```python
from build123d import *

# Parameters (mm, degrees)
SKETCH1_W           = 72
SKETCH1_H           = 47
SKETCH1_W_2         = 5
SKETCH1_H_2         = 13.68224698
SKETCH1_H_3         = 13
BOSS_EXTRUDE1_DEPTH = 5
SKETCH3_W           = 14.035397612
SKETCH3_H           = 7.623801165
BOSS_EXTRUDE3_DEPTH = 5
SKETCH5_W           = 14.035397612
SKETCH5_H           = 7.623801165
BOSS_EXTRUDE4_DEPTH = 5
SKETCH4_R           = 1.799999998
CUT_EXTRUDE1_DEPTH  = 95
SKETCH6_W           = 72
SKETCH6_H           = 5
BOSS_EXTRUDE5_DEPTH = 21
SKETCH8_W           = 114.485355007
SKETCH8_H           = 45.141194617
CUT_EXTRUDE2_DEPTH  = 4.5
SKETCH9_W           = 62
SKETCH9_H           = 5
CUT_EXTRUDE3_DEPTH  = 4.5


with BuildPart() as part:
    # Sketch1 → Boss-Extrude1 (new body)
    with BuildSketch(Plane(origin=(0, 0, 0), x_dir=(1, 0, 0), z_dir=(0, 1, 0))):
        with Locations((36, -23.5)):
            Rectangle(SKETCH1_W, SKETCH1_H)
        with Locations((69.5, 6.84112349)):
            Rectangle(SKETCH1_W_2, SKETCH1_H_2)
        with Locations((2.5, 6.5)):
            Rectangle(SKETCH1_W_2, SKETCH1_H_3)
    extrude(amount=BOSS_EXTRUDE1_DEPTH)

    # Sketch3 → Boss-Extrude3 (add)
    with BuildSketch(Plane(origin=(72, 0, 0), x_dir=(0, 0, -1), z_dir=(1, 0, 0))):
        with Locations((6.664548174, 1.188099417)):
            Rectangle(SKETCH3_W, SKETCH3_H)
    extrude(amount=-BOSS_EXTRUDE3_DEPTH)

    # Sketch5 → Boss-Extrude4 (add)
    with BuildSketch(Plane.ZY):
        with Locations((-6.664548174, 1.188099417)):
            Rectangle(SKETCH5_W, SKETCH5_H)
    extrude(amount=-BOSS_EXTRUDE4_DEPTH)

    # Sketch4 → Cut-Extrude1 (cut)
    with BuildSketch(Plane(origin=(72, 0, 0), x_dir=(0, 0, -1), z_dir=(1, 0, 0))):
        with Locations((4.182640247, 1.972422216)):
            Circle(SKETCH4_R)
    extrude(amount=-CUT_EXTRUDE1_DEPTH, mode=Mode.SUBTRACT)

    # Sketch6 → Boss-Extrude5 (add)
    with BuildSketch(Plane.XY.offset(47)):
        with Locations((36, 2.5)):
            Rectangle(SKETCH6_W, SKETCH6_H)
    extrude(amount=BOSS_EXTRUDE5_DEPTH)

    # Sketch8 → Cut-Extrude2 (cut)
    with BuildSketch(Plane(origin=(0, 0, -13.68224698), x_dir=(-1, 0, 0), z_dir=(0, 0, -1))):
        with Locations((-40.6465034, -1.597733879)):
            Rectangle(SKETCH8_W, SKETCH8_H)
    extrude(amount=-CUT_EXTRUDE2_DEPTH, mode=Mode.SUBTRACT)

    # Sketch9 → Cut-Extrude3 (cut)
    with BuildSketch(Plane(origin=(0, 0, 0), x_dir=(-1, 0, 0), z_dir=(0, 0, -1))):
        with Locations((-36, 2.5)):
            Rectangle(SKETCH9_W, SKETCH9_H)
    extrude(amount=-CUT_EXTRUDE3_DEPTH, mode=Mode.SUBTRACT)


solid = part.part
```
Work out the finished part from the listing and answer in its coordinate system (mm). A direction names the side the tool comes from. Give positions to 0.01 mm unless a question says otherwise; leave off trailing zeros. Order: outer loops, then holes, each group sorted by start corner. A loop starts at its lowest first (then second) coordinate and runs counter-clockwise, first axis right, second up.
1. For faces 4 (the flat face through (35, 3, 68)), 5 (the flat face through (35, 0, 34)), 6 (the flat face through (36, 3, 4.5)), determine the directions among +Z, -Z, +X, -X, +Y, -Y from which every point of the face is accessible in a straight line to the end or side of a thin tool.
Result sheet:
face 4: +Z, +X, -X, +Y, -Y
face 5: +Z, +X, -X, -Y
face 6: -Z, +Y, -Y
2. Section A-A, the plane y = -1.5 is taken. Determine the outline of the cut face in (x, z), and give its area (3 significant figures).
Result sheet:
outline: (0, -9.18) - (5, -9.18) - (5, 0.35) - (0, 0.35) - close; (67, -9.18) - (72, -9.18) - (72, 0.35) - (67, 0.35) - close
area: 95.4 mm2
3. Section B-B, the plane x = 6 is taken. Determine the outline of the cut face in (y, z).
Result sheet:
outline: (0, 4.5) - (5, 4.5) - (5, 68) - (0, 68) - close
4. Section C-C, the plane z = 7 is taken. Determine the outline of the cut face in (x, y).
Result sheet:
outline: (0, 0) - (72, 0) - (72, 5) - (0, 5) - close
5. Straight lines are drawn through the part: L1, parallel to Y at x = 20, z = 19; L2, parallel to Z at x = 43, y = 4.5; L3, parallel to Z at x = 4.5, y = 3.5. For each, find the intervals that lie inside material, in ascending order.
Result sheet:
L1: y = 0 to 5
L2: z = 4.5 to 68
L3: z = -9.18 to -5.13, -3.23 to 68
6. Each of these flat-tipped pins is pushed along its axis until it touches: P1, Ø1.3, axis at x = 70, y = -1.5, coming from the +Z side; P2, Ø1, axis at x = 38.5, y = -2, coming from the -Z side; P3, Ø2, axis at x = 35, z = 42.5, coming from the -Y side. Where does it stop, or does it pass through?
Result sheet:
P1: stops at z = 0.35
P2: passes through
P3: stops at y = 0
7. The mould has two halves that part along Z. Classify faces 1 (the flat face through (67, 1, -2)), 2 (the cylindrical face through (69.54, 2.51, -5.9)), 3 (the flat face through (2, -1, 0.353)): released by +Z, released by -Z, zero draft, split by the parting line, or undercut.
Result sheet:
face 1: zero draft
face 2: undercut
face 3: released by +Z
